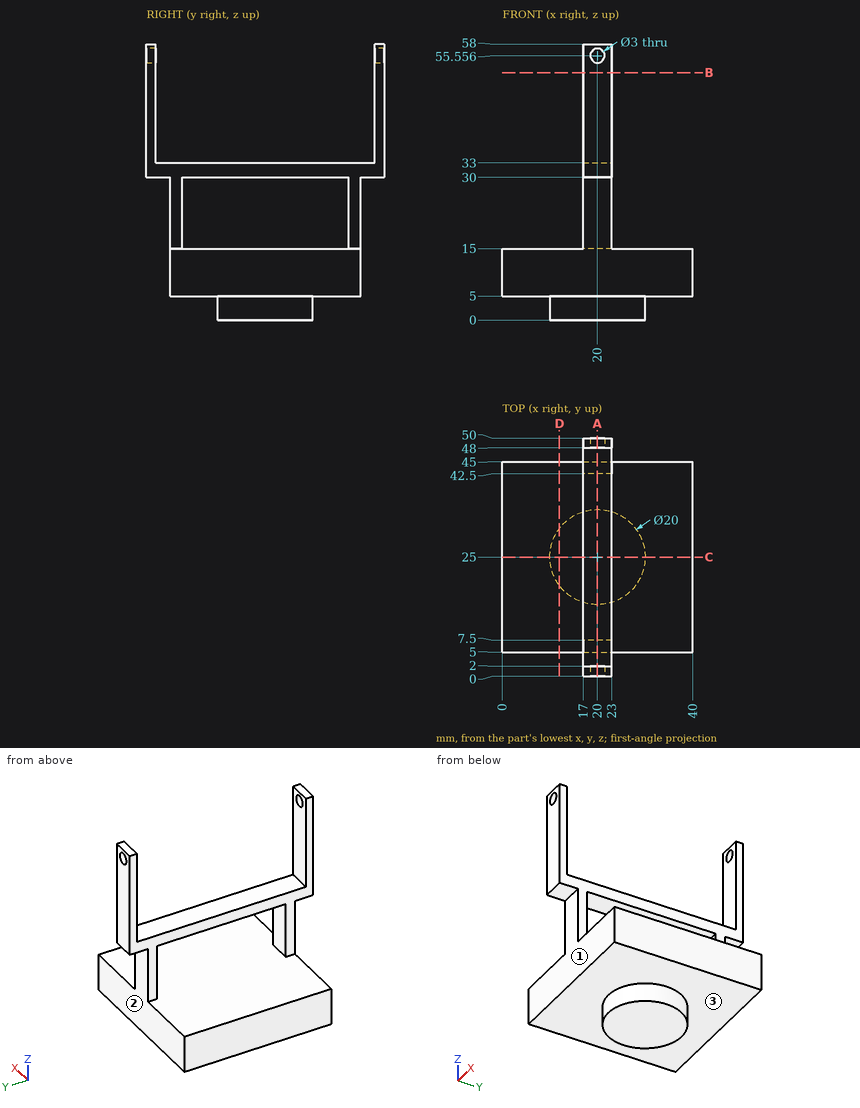
Here's the drawing with two shaded views (mm, measured from the low corner). I have some questions. A direction names the side the tool comes from. Give positions to 0.01 mm unless a question says otherwise; leave off trailing zeros. Order: outer loops, then holes, each group sorted by start corner. A loop starts at its lowest first (then second) coordinate and runs counter-clockwise, first axis right, second up. Notation, with made-up numbers: (8, 25.25) -> (58, 25.25) arc R32 cw to (58, 54.25) -> close; hole circle Ø10 at (28, 83.25). An arc over 180 degrees is marked (long way). One line per item, written item: value. Start each with the question number.
1. Will these pins go through, and if not, where does the flat tip stop? pin 1 Ø20 at (x, z) = (28.5, 20) entering from -Y; pin 2 Ø6.5 at (x, z) = (19.5, 19.5) entering from +Y; pin 3 Ø13 at (y, z) = (18.5, 27) entering from -X.
2. Imagine slicing it at C-C, the plane y = 25. List the corners of the cut face in (x, z) for me, plus the area to 3 significant figures.
3. Imagine slicing it at A-A, the plane x = 20. List the corners of the cut face in (y, z) for me (1 decimal).
4. For the marked faces 1, 2 and 3, which set-ups out of +Z, -Z, +X, -X, +Y, -Y let a thin tool reach every point of the face, with its end or its side?
5. Imagine slicing it at B-B, the plane z = 52. List the corners of the cut face in (x, y) for me, plus the area to 3 significant figures.
6. Imagine slicing it at D-D, the plane x = 12. List the corners of the cut face in (y, z) for me, plus the area to 3 significant figures.
7. I need wall thicknesses on probe 1 along Y at (x, z) = (18, 44.5); probe 2 along Y at (x, z) = (22, 19); probe 3 along X at (y, z) = (7, 29). Which ranges of each line are inside material? Lowest first, please. Write a range as from..to.
Values follow:
1. pin 1: stops at y = 5
1. pin 2: stops at y = 45
1. pin 3: stops at x = 17
2. outline: (0, 5) -> (10, 5) -> (10, 0) -> (30, 0) -> (30, 5) -> (40, 5) -> (40, 15) -> (0, 15) -> close; (17, 30) -> (23, 30) -> (23, 33) -> (17, 33) -> close
2. area: 518 mm2
3. outline: (0, 30) -> (5, 30) -> (5, 5) -> (15, 5) -> (15, 0) -> (35, 0) -> (35, 5) -> (45, 5) -> (45, 30) -> (50, 30) -> (50, 54.1) -> (48, 54.1) -> (48, 33) -> (2, 33) -> (2, 54.1) -> (0, 54.1) -> close; (0, 57.1) -> (2, 57.1) -> (2, 58) -> (0, 58) -> close; (48, 57.1) -> (50, 57.1) -> (50, 58) -> (48, 58) -> close; hole (7.5, 15) -> (42.5, 15) -> (42.5, 30) -> (7.5, 30) -> close
4. face 1: -Z, +X, -X, -Y
4. face 2: -Z, +X, -X, +Y
4. face 3: -Z
5. outline: (17, 0) -> (23, 0) -> (23, 2) -> (17, 2) -> close; (17, 48) -> (23, 48) -> (23, 50) -> (17, 50) -> close
5. area: 24.0 mm2
6. outline: (5, 5) -> (19, 5) -> (19, 0) -> (31, 0) -> (31, 5) -> (45, 5) -> (45, 15) -> (5, 15) -> close
6. area: 460 mm2
7. probe 1: y = 0..2, 48..50
7. probe 2: y = 5..7.5, 42.5..45
7. probe 3: x = 17..23
